Geometry check sheet. Reference: drawing and pictorial views, mm from the part's lowest x, y, z. A direction names the side the tool comes from. Give positions to 0.01 mm unless a question says otherwise; leave off trailing zeros. Order: outer loops, then holes, each group sorted by start corner. A loop starts at its lowest first (then second) coordinate and runs counter-clockwise, first axis right, second up. Notation, with made-up numbers: M 4,73 L 42,73 A33 ccw 42,104 Z; hole C 21,30 d10. An arc over 180 degrees is marked long. Use CSV: the item, a comma, the result in double quotes. Start each with the question number.
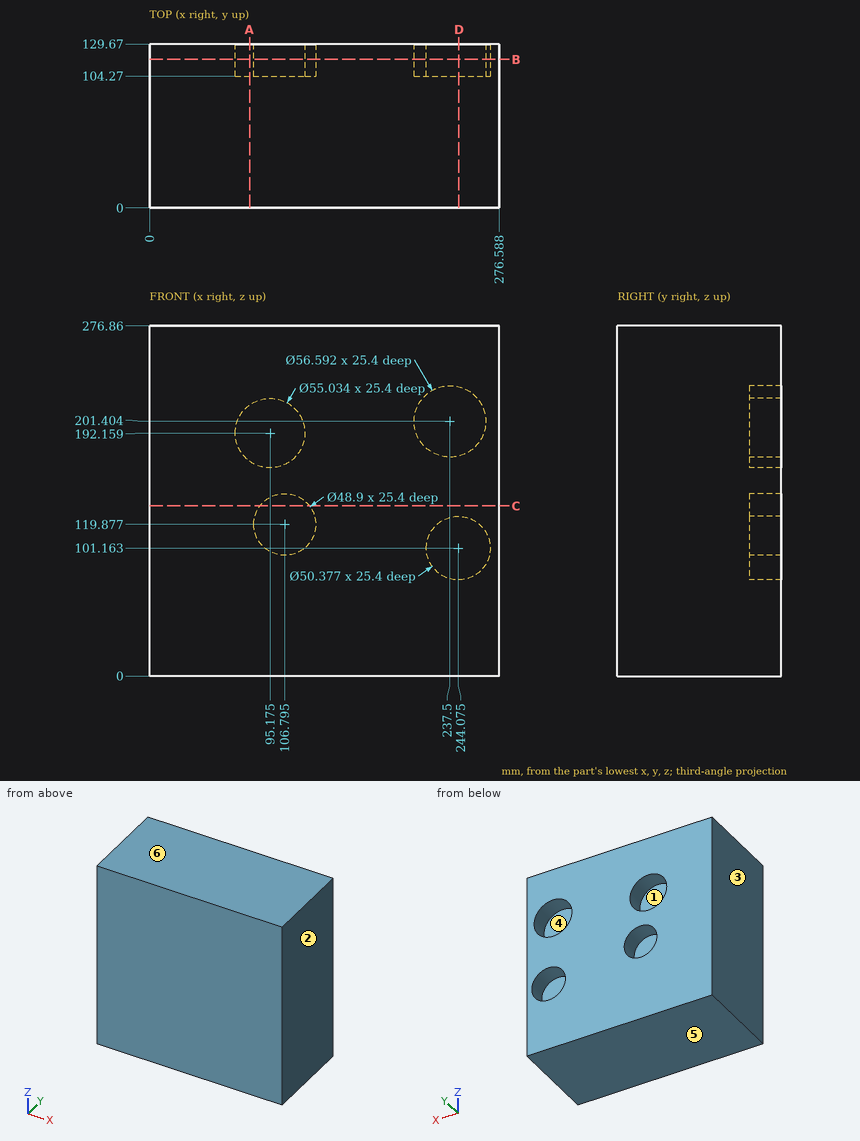
(1) Sectioned sample at A-A on x = 79. Record the cut outline in (y, z).
(2) Thickness scan on line 1 (X direction, y = 115, z = 118) (1 decimal); line 2 (X direction, y = 118, z = 220.5); line 3 (Y direction, x = 113.5, z = 133). Record the ranges inside material, lowest first.
(3) Sectioned sample at C-C on z = 134.5. Record the cut outline in (x, y).
(4) Draft check along Z on the marked faces 3, 4, 5 and 6. Enter one of: +Z half, -Z half, draft (parallel to the pull), parting line (faces both ways), or undercut.
(5) Go/stop test with a flat-tipped pin: P1, Ø2, axis at x = 80.5, z = 205.5, coming from the +Y side. Record where the tip stops, or that it passes through.
(6) Access from +Z, -Z, +X, -X, +Y, -Y to the whole of each face (thin tool, end or side, straight path). Record for the marked faces 1 and 2.
(7) Sectioned sample at D-D on x = 244.5. Record the cut outline in (y, z), then the cut area to 3 significant figures.
(8) Sectioned sample at B-B on y = 117.5. Give the number of separate pieces and of enclosed holes in the cut face, then the cut area to 3 significant figures.
Responses:
1,outline,"M 0,0 L 129.67,0 L 129.67,169.9 L 104.27,169.9 L 104.27,214.42 L 129.67,214.42 L 129.67,276.86 L 0,276.86 Z"
2,line 1,"0 to 82.4, 131.2 to 225.3, 262.8 to 276.6"
2,line 2,"0 to 216.62, 258.38 to 276.59"
2,line 3,"0 to 104.27"
3,outline,"M 0,0 L 276.59,0 L 276.59,129.67 L 126.39,129.67 L 126.39,104.27 L 87.2,104.27 L 87.2,129.67 L 0,129.67 Z"
4,face 3,"draft"
4,face 4,"undercut"
4,face 5,"-Z half"
4,face 6,"+Z half"
5,P1,"y = 104.27"
6,face 1,"+Y"
6,face 2,"+Z, -Z, +X, +Y, -Y"
7,outline,"M 0,0 L 129.67,0 L 129.67,75.98 L 104.27,75.98 L 104.27,126.35 L 129.67,126.35 L 129.67,173.99 L 104.27,173.99 L 104.27,228.82 L 129.67,228.82 L 129.67,276.86 L 0,276.86 Z"
7,area,"33,200 mm2"
8,separate pieces,"1"
8,enclosed holes,"4"
8,area,"67,800 mm2"
